The model under review builds one solid part; all positions refer to its coordinate system, in mm. A direction names the side the tool comes from. Round coordinates to 2 decimals unless told otherwise and drop trailing zeros. Write each loop counter-clockwise with the first axis right and the second up, starting at its lowest first coordinate (ties: lowest second). Pieces come first, ordered by that corner, then holes. Notation, with made-up numbers: M -18,-33 L -8,-33 A21 cw -8,1 Z; hole C 62,58 d10. An arc over 180 degrees is marked long. Write item = value, one per line. Start each with the question number.
Item 1: To check wall thickness, follow line 1 along Y through (x, z) = (0, 1.7); line 2 along X through (y, z) = (-1.75, 1.5); line 3 along Y through (x, z) = (-23.5, 1.9). State the ranges of each line that lie inside material, in increasing order.
Item 2: The part is to be moulded in two halves that separate along Y. For faces 3 (the flat face through (13, 0, 2)), 4 (the flat face through (-9, 10, 3.175)), 5 (the cylindrical face through (-3, 0, 2)), 6 (the cylindrical face through (14.297, 13.986, 1.565)), say which applies: +Y half, -Y half, draft (parallel to the pull), parting line (faces both ways), or undercut.
Item 3: Take a section at C-C, the plane y = 9.5. Give the boundary of the cut face in (x, z) (3 decimals), plus the area to 3 significant figures.
Item 4: Take a section at A-A, the plane z = 2.45. Give the boundary of the cut face in (x, y).
Item 5: Tool access review of faces 1 (the flat face through (-22, 0, 2)), 2 (the flat face through (-36.842, 10, 2)): name each direction out of +Z, -Z, +X, -X, +Y, -Y from which nothing blocks a thin tool from reaching the whole face with its end or side.
Item 6: For pin 1 Ø1 at (x, z) = (-22, 1) entering from -Y, flat-tipped, find the tip position at first contact; note if it passes through.
Item 7: Take a section at D-D, the plane x = 7. Give the boundary of the cut face in (y, z) (3 decimals), plus the area to 3 significant figures.
Item 8: Take a section at B-B, the plane y = 1.5. Give the boundary of the cut face in (x, z) (3 decimals).
from build123d import *

# Parameters (mm, degrees)
SKETCH1_R           = 3
BOSS_EXTRUDE1_DEPTH = 3.175


with BuildPart() as part:
    # Sketch1 → Boss-Extrude1 (new body)
    with BuildSketch(Plane.XY):
        with BuildLine():
            ThreePointArc((-6, 0), (0, -6), (6, 0))
            Line((6, 0), (20, 0))
            ThreePointArc((20, 0), (14.142135624, 14.142135624), (0, 20))
            Line((0, 20), (-36.84213525, 20))
            Line((-36.84213525, 20), (-36.84213525, 0))
            Line((-36.84213525, 0), (-6, 0))
        make_face()
        Circle(SKETCH1_R, mode=Mode.SUBTRACT)
    extrude(amount=BOSS_EXTRUDE1_DEPTH)


solid = part.part
Response values:
q1.line_1 = -6 to -3, 3 to 20
q1.line_2 = -5.74 to -2.44, 2.44 to 5.74
q1.line_3 = 0 to 20
q2.face_3 = -Y half
q2.face_4 = draft
q2.face_5 = undercut
q2.face_6 = +Y half
q3.outline = M -36.842,0 L 17.6,0 L 17.6,3.175 L -36.842,3.175 Z
q3.area = 173 mm2
q4.outline = M -36.84,0 L -6,0 A6 ccw 6,0 L 20,0 A20 ccw 0,20 L -36.84,20 Z; hole C 0,0 d6
q5.face_1 = +Z, -Z, -X, -Y
q5.face_2 = +Z, -Z, -X, +Y, -Y
q6.pin_1 = 0
q7.outline = M 0,0 L 18.735,0 L 18.735,3.175 L 0,3.175 Z
q7.area = 59.5 mm2
q8.outline = M -36.842,0 L -2.598,0 L -2.598,3.175 L -36.842,3.175 Z; M 2.598,0 L 19.944,0 L 19.944,3.175 L 2.598,3.175 Z
